```python
from build123d import *

# Parameters (mm, degrees)
F0_R     = 39.700031
F0_R_2   = 26.502297
F1_DEPTH = 46.736
F3_DEPTH = 10.668
F5_DEPTH = 5.588


with BuildPart() as f1:
    # F0 (on Top) → F1 (new body)
    with BuildSketch(Plane.XY):
        with Locations((39.700031, 0)):
            Circle(F0_R)
        with Locations((39.700031, 0)):
            Circle(F0_R_2, mode=Mode.SUBTRACT)
    extrude(amount=F1_DEPTH)

    # F2 (on face) → F3 (join)
    with BuildSketch(Plane(origin=(0, 0, 0), x_dir=(1, 0, 0), z_dir=(0, 0, -1))):
        with BuildLine():
            Line((-63.262849, -35.048185), (21.052854, -35.048185))
            ThreePointArc((21.052854, -35.048185), (0, 0), (21.052854, 35.048185))
            Line((21.052854, 35.048185), (-63.262849, 35.048185))
            Line((-63.262849, 35.048185), (-63.262849, -35.048185))
        make_face()
    extrude(amount=-F3_DEPTH)

    # F4 (on Front) → F5 (join, symmetric)
    with BuildSketch(Plane.XZ):
        Polygon((4.870512, 38.895372), (-47.924407, 7.358584), (4.870512, 6.657766), align=None)
    extrude(amount=F5_DEPTH, both=True)


solid = f1.part
```
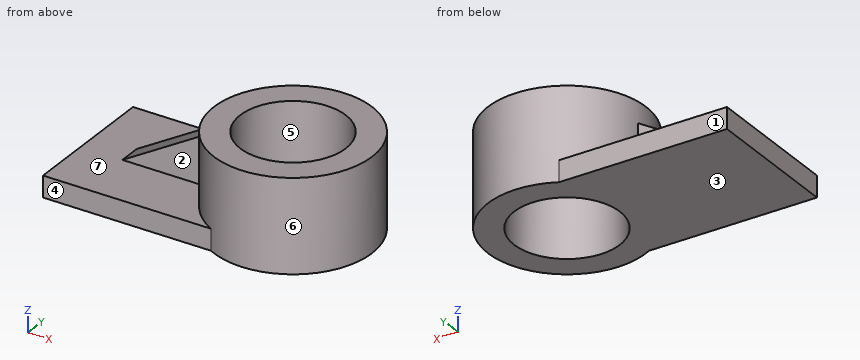
Model file for the job. Use its own axes, mm. Face numbers are marked on the shaded views. A direction names the side the tool comes from. Coordinates: 2 decimals unless noted, no trailing zeros. Loops run counter-clockwise (first coordinate to the right, second up) from the corner with the lowest first, then second, coordinate; pieces in that order, holes last. Notation, with made-up numbers: (-4.75, 33.25) - (21.25, 33.25) arc R18 ccw to (21.25, 56.25) - close; hole circle Ø4 at (63.25, 47). An arc over 180 degrees is marked (long way). Write item = value, one per line. Start each with the question number.
Item 1: Saw through at C-C, the plane y = 0. List the corners of the cut face in (x, z), then the cut area to 3 significant figures.
Item 2: Pull direction Y, two halves, no side cores. Call the marked faces 4, 5, 6 and 7: +Y half, -Y half, draft (parallel to the pull), parting line (faces both ways), or undercut.
Item 3: Saw through at D-D, the plane x = -4. List the corners of the cut face in (y, z).
Item 4: 3-axis set-ups, long thin cutter, end or side, ignore diameter. For the marked faces 1, 2 and 3: which of +Z, -Z, +X, -X, +Y, -Y reach the whole face in a straight line?
Item 5: Saw through at A-A, the plane x = 33. List the corners of the cut face in (y, z), then the cut area to 3 significant figures.
Item 6: Drop flat-ended pins along their axis: pin 1 Ø6 at (y, z) = (4.5, 37.5) entering from -X; pin 2 Ø1 at (y, z) = (-5.5, 19) entering from +X; pin 3 Ø10 at (x, z) = (48, 18.5) entering from -Y. Give the stop position or say it passes through.
Item 7: Wall check: probe 1 along Z at (x, y) = (3.5, 16.5); probe 2 along Y at (x, z) = (-26, 2.5); probe 3 along X at (y, z) = (23, 33). Give the ranges that are in metal, low to high. Write a range as [from, to].
Item 8: Saw through at B-B, the plane z = 8.5. List the corners of the cut face in (x, y), then the cut area to 3 significant figures.
Answers:
q1.outline = (-63.26, 0) - (13.2, 0) - (13.2, 46.74) - (0, 46.74) - (0, 35.99) - (-42.38, 10.67) - (-63.26, 10.67) - close; (66.2, 0) - (79.4, 0) - (79.4, 46.74) - (66.2, 46.74) - close
q1.area = 2,450 mm2
q2.face_4 = -Y half
q2.face_5 = undercut
q2.face_6 = parting line
q2.face_7 = draft
q3.outline = (-35.05, 0) - (35.05, 0) - (35.05, 10.67) - (5.59, 10.67) - (5.59, 33.6) - (-5.59, 33.6) - (-5.59, 10.67) - (-35.05, 10.67) - close
q4.face_1 = +Z, -Z, -X, +Y
q4.face_2 = +Z, -X, -Y
q4.face_3 = -Z, +X, -X, +Y, -Y
q5.outline = (-39.13, 0) - (-25.64, 0) - (-25.64, 46.74) - (-39.13, 46.74) - close; (25.64, 0) - (39.13, 0) - (39.13, 46.74) - (25.64, 46.74) - close
q5.area = 1,260 mm2
q6.pin_1 = -2.49
q6.pin_2 = 79.08
q6.pin_3 = -39.56
q7.probe_1 = [0, 10.67]
q7.probe_2 = [-35.05, 35.05]
q7.probe_3 = [7.34, 26.53], [52.87, 72.06]
q8.outline = (-63.26, -35.05) - (21.05, -35.05) arc R39.7 ccw (long way) to (21.05, 35.05) - (-63.26, 35.05) - close; hole circle Ø53 at (39.7, 0)
q8.area = 7,600 mm2
